Check sheet for the drawn part. Datum: minimum x, y, z corner. Units: mm. A direction names the side the tool comes from. Give positions to 0.01 mm unless a question says otherwise; leave off trailing zeros. Write each loop counter-clockwise with the first axis right and the second up, starting at its lowest first coordinate (ties: lowest second). Pieces come first, ordered by that corner, then holes. Notation, with made-up numbers: M 43,-5 L 64,-5 A10 ccw 64,6 Z; hole C 68,-18.5 d4. An arc over 180 degrees is marked long. Use CSV: the item, a comma, the result in double quotes. Start each with the question number.
1. Depth check by flat-ended pin: P1, Ø3, axis at x = 47.5, y = 16, coming from the +Z side; P2, Ø4, axis at x = 6.5, y = 6.5, coming from the -Z side; P3, Ø6, axis at y = 46.5, z = 2, coming from the -X side (1 decimal). Enter the tip coordinate at first touch or a pass-through.
2. Scan lines: line 1 (X direction, y = 29, z = 12.25); line 2 (Y direction, x = 35, z = 7.25). Record each from-to range of solid material in increasing order.
3. Access from +Z, -Z, +X, -X, +Y, -Y to the whole of each face (thin tool, end or side, straight path). Record for the marked faces 4, 5 and 6.
4. Mould release check, pull along Y, two halves, no side actions. Record for the marked faces 1, 2 and 3: +Y half, -Y half, draft (parallel to the pull), parting line (faces both ways), or undercut.
5. Cross-section at C-C, the plane y = 39.5. Enter the section's corners in (x, z).
6. Cross-section at B-B, the plane z = 12.75. Enter the section's corners in (x, y).
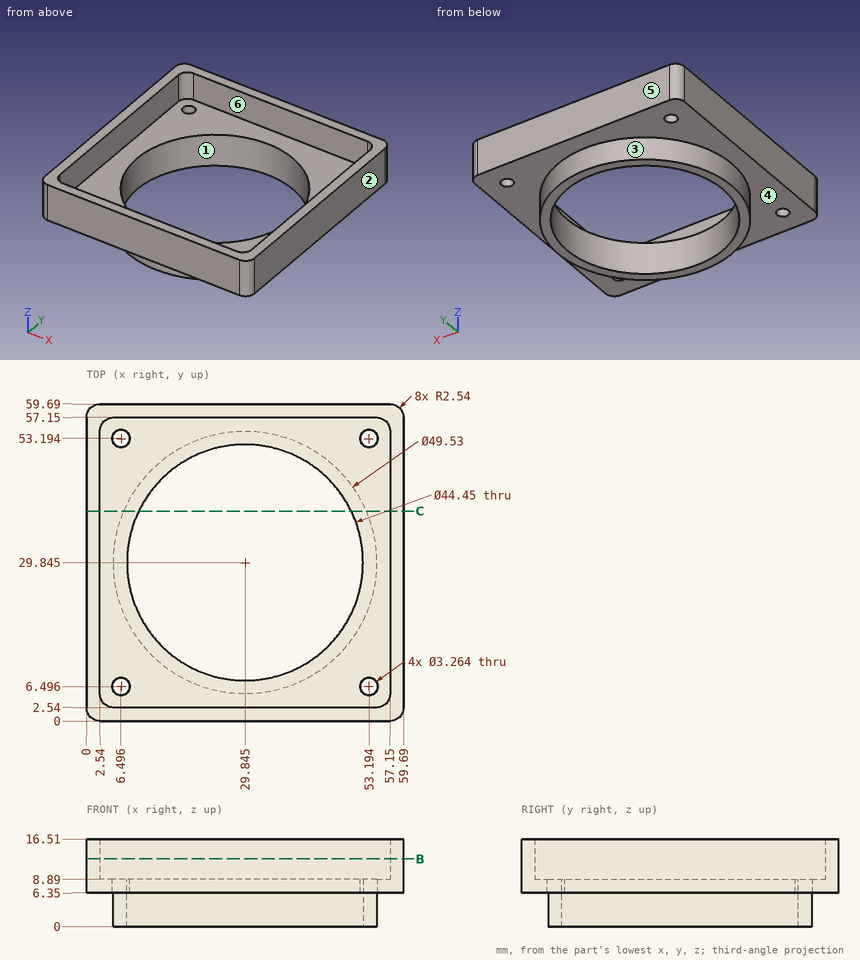
Worked answers:
1,P1,"stops at z = 8.89"
1,P2,"stops at z = 6.35"
1,P3,"stops at x = 9.2"
2,line 1,"x = 0 to 2.54, 57.15 to 59.69"
2,line 2,"y = 0 to 8.23, 51.46 to 59.69"
3,face 4,"-Z"
3,face 5,"+Z, -Z, +X, -X, +Y"
3,face 6,"+Z"
4,face 1,"undercut"
4,face 2,"draft"
4,face 3,"parting line"
5,outline,"M 0,6.35 L 7.04,6.35 L 7.04,0 L 9.83,0 L 9.83,8.89 L 2.54,8.89 L 2.54,16.51 L 0,16.51 Z; M 49.86,0 L 52.65,0 L 52.65,6.35 L 59.69,6.35 L 59.69,16.51 L 57.15,16.51 L 57.15,8.89 L 49.86,8.89 Z"
6,outline,"M 0,2.54 A2.54 ccw 2.54,0 L 57.15,0 A2.54 ccw 59.69,2.54 L 59.69,57.15 A2.54 ccw 57.15,59.69 L 2.54,59.69 A2.54 ccw 0,57.15 Z; hole M 2.54,5.08 A2.54 ccw 5.08,2.54 L 54.61,2.54 A2.54 ccw 57.15,5.08 L 57.15,54.61 A2.54 ccw 54.61,57.15 L 5.08,57.15 A2.54 ccw 2.54,54.61 Z"
